from build123d import *

# Parameters (mm, degrees)
SKETCH1_W           = 20
SKETCH1_H           = 23
BOSS_EXTRUDE1_DEPTH = 10
CUT_EXTRUDE1_DEPTH  = 7
SKETCH4_R           = 4.55
CUT_EXTRUDE6_DEPTH  = 7
SKETCH9_W           = 14.55
SKETCH9_H           = 7
CUT_EXTRUDE8_DEPTH  = 1.5
SKETCH10_W          = 15.291428019
SKETCH10_H          = 6
CUT_EXTRUDE9_DEPTH  = 5.5
SKETCH11_R          = 1
CUT_EXTRUDE10_DEPTH = 5.5


with BuildPart() as part:
    # Sketch1 → Boss-Extrude1 (new body)
    with BuildSketch(Plane(origin=(0, 0, 0), x_dir=(1, 0, 0), z_dir=(0, 1, 0))):
        Rectangle(SKETCH1_W, SKETCH1_H)
    extrude(amount=BOSS_EXTRUDE1_DEPTH)

    # Sketch3 → Cut-Extrude1 (cut)
    with BuildSketch(Plane(origin=(0, 10, 0), x_dir=(1, 0, 0), z_dir=(0, 1, 0))):
        Polygon((0, -11.5), (-7, -11.5), (-7, 8.5), (7, 8.5), (7, -11.5), align=None)
    extrude(amount=-CUT_EXTRUDE1_DEPTH, mode=Mode.SUBTRACT)

    # Sketch4 → Cut-Extrude6 (cut)
    with BuildSketch(Plane(origin=(10, 0, 0), x_dir=(0, 0, -1), z_dir=(1, 0, 0))):
        with Locations((-1.5, 10)):
            Circle(SKETCH4_R)
    extrude(amount=-CUT_EXTRUDE6_DEPTH, mode=Mode.SUBTRACT)

    # Sketch9 → Cut-Extrude8 (cut)
    with BuildSketch(Plane.ZY.offset(-7)):
        with Locations((1.5, 6.5)):
            Rectangle(SKETCH9_W, SKETCH9_H)
    extrude(amount=-CUT_EXTRUDE8_DEPTH, mode=Mode.SUBTRACT)

    # Sketch10 → Cut-Extrude9 (cut)
    with BuildSketch(Plane.ZY.offset(10)):
        with Locations((3.854285991, 7)):
            Rectangle(SKETCH10_W, SKETCH10_H)
    extrude(amount=-CUT_EXTRUDE9_DEPTH, mode=Mode.SUBTRACT)

    # Sketch11 → Cut-Extrude10 (cut)
    with BuildSketch(Plane.XZ):
        with Locations(Location((2.88, 9.5, 0), (0, 0, 270))):
            Circle(SKETCH11_R)
        with Locations(Location((2.88, -6.5, 0), (0, 0, 270))):
            Circle(SKETCH11_R)
    extrude(amount=-CUT_EXTRUDE10_DEPTH, mode=Mode.SUBTRACT)


solid = part.part
Work out the finished part from the listing and answer in its coordinate system (mm). A direction names the side the tool comes from. Give positions to 0.01 mm unless a question says otherwise; leave off trailing zeros. Order: outer loops, then holes, each group sorted by start corner. A loop starts at its lowest first (then second) coordinate and runs counter-clockwise, first axis right, second up. Notation, with made-up numbers: (11.5, -6.5) -> (49.5, -6.5) arc R28 cw to (49.5, 27.5) -> close; hole circle Ø8 at (40.25, 19). An arc over 180 degrees is marked (long way). One line per item, written item: value.
Item 1: Flat-ended cylindrical pins translate along their axes: P1, Ø0.8, axis at y = 6, z = 10, coming from the -X side; P2, Ø3.5, axis at x = -8, y = 8.5, coming from the +Z side; P3, Ø5.5, axis at x = 0.5, y = 8, coming from the +Z side. Find the tip coordinate at first contact, or state that the pin passes through.
Answer sheet:
P1: x = 7
P2: z = -3.79
P3: z = -8.5
Item 2: Find section C-C, the plane y = 8.5. Give the vertices of the cut face in (x, z) (3 decimals), plus the area to 3 significant figures.
Answer sheet:
outline: (-10, -11.5) -> (10, -11.5) -> (10, -2.796) -> (8.5, -2.796) -> (8.5, -5.775) -> (7, -5.775) -> (7, -8.5) -> (-7, -8.5) -> (-7, -3.791) -> (-10, -3.791) -> close; (7, 8.775) -> (8.5, 8.775) -> (8.5, 5.796) -> (10, 5.796) -> (10, 11.5) -> (7, 11.5) -> close
area: 99.4 mm²
Item 3: Straight lines are drawn through the part: probe 1 along X at (y, z) = (1.15, -6.5); probe 2 along X at (y, z) = (3.75, 8.5); probe 3 along Y at (x, z) = (-6, 7). For each, find the intervals that lie inside material, in ascending order.
Answer sheet:
probe 1: -10 to 1.88, 3.88 to 10
probe 2: -10 to -7, 8.5 to 10
probe 3: 0 to 3
Item 4: A tool of negligible diameter and unlimited length cuts with its end or side. For faces 4 (the flat face through (7, 7, -7)), 5 (the flat face through (0, 5, -11.5)), 6 (the flat face through (-9, 4, 4)), from which of +Z, -Z, +X, -X, +Y, -Y can it reach the whole face along a straight path? Write none if from no direction.
Answer sheet:
face 4: +Z, +Y
face 5: -Z, +X, -X, +Y, -Y
face 6: +Z, -X, +Y
Item 5: Determine the mould class of faces 1 (the flat face through (8.5, 5, 1)), 2 (the flat face through (-9, 7, -3.791)), 3 (the flat face through (10, 5, 0)) for opening direction Z: released by +Z, released by -Z, zero draft, split by the parting line, or undercut.
Answer sheet:
face 1: undercut
face 2: released by +Z
face 3: zero draft
Item 6: Find section D-D, the plane x = 8. Give the vertices of the cut face in (y, z) (3 decimals), plus the area to 3 significant figures.
Answer sheet:
outline: (0, -11.5) -> (10, -11.5) -> (10, -5.775) -> (3, -5.775) -> (3, 8.775) -> (10, 8.775) -> (10, 11.5) -> (0, 11.5) -> close
area: 128 mm²
Item 7: Find section A-A, the plane x = 2.88. Give the vertices of the cut face in (y, z), plus the area to 3 significant figures.
Answer sheet:
outline: (0, -11.5) -> (10, -11.5) -> (10, -8.5) -> (3, -8.5) -> (3, -7.5) -> (0, -7.5) -> close; (0, -5.5) -> (3, -5.5) -> (3, 8.5) -> (0, 8.5) -> close; (0, 10.5) -> (3, 10.5) -> (3, 11.5) -> (0, 11.5) -> close
area: 78.0 mm²
Item 8: Find section B-B, the plane z = -6.5. Give the vertices of the cut face in (x, y), plus the area to 3 significant figures.
Answer sheet:
outline: (-10, 0) -> (1.88, 0) -> (1.88, 3) -> (-7, 3) -> (-7, 10) -> (-10, 10) -> close; (3.88, 0) -> (10, 0) -> (10, 10) -> (7, 10) -> (7, 3) -> (3.88, 3) -> close
area: 96.0 mm²
